CAD build for the part. Positions are in the model's coordinates, mm. Give positions to 0.01 mm unless a question says otherwise; leave off trailing zeros. Loops run counter-clockwise (first coordinate to the right, second up) from the corner with the lowest first, then second, coordinate; pieces in that order, holes last.
```python
from build123d import *

# Parameters (mm, degrees)
SKETCH_1_W             = 209.2
SKETCH_1_H             = 110
SM_BASE_FLANGE_1_DEPTH = 3.6
CUT_EXTRUDE_1_REACH    = 238.384
SKETCH_2_W             = 3.6
SKETCH_2_H             = 22
SKETCH_2_W_2           = 24
SKETCH_2_H_2           = 3.6
SKETCH_2_W_3           = 26
CUT_EXTRUDE_2_REACH    = 238.384
SKETCH_3_R             = 1.6


# Sheet-metal steps are written as plain solids
with BuildPart() as part:
    # Sketch 1 → Базовая кромка1 (new body)
    with BuildSketch(Plane.XY):
        with Locations((104.6, 55)):
            Rectangle(SKETCH_1_W, SKETCH_1_H)
    extrude(amount=-SM_BASE_FLANGE_1_DEPTH)

    # Sketch 2 → Вырез-Вытянуть1 (cut, up to next)
    with BuildSketch(Plane.XY, mode=Mode.PRIVATE) as cut_extrude_1_sk1:
        with Locations((1.8, 23)):
            Rectangle(SKETCH_2_W, SKETCH_2_H)
    cut_extrude_1_tool1 = extrude(cut_extrude_1_sk1.sketch, amount=-CUT_EXTRUDE_1_REACH, mode=Mode.PRIVATE) & part.part
    # Sketch 2 → Вырез-Вытянуть1 (cut, up to next)
    with BuildSketch(Plane.XY, mode=Mode.PRIVATE) as cut_extrude_1_sk2:
        with Locations((35.6, 1.8)):
            Rectangle(SKETCH_2_W_2, SKETCH_2_H_2)
    cut_extrude_1_tool2 = extrude(cut_extrude_1_sk2.sketch, amount=-CUT_EXTRUDE_1_REACH, mode=Mode.PRIVATE) & part.part
    # Sketch 2 → Вырез-Вытянуть1 (cut, up to next)
    with BuildSketch(Plane.XY, mode=Mode.PRIVATE) as cut_extrude_1_sk3:
        with Locations((207.4, 87)):
            Rectangle(SKETCH_2_W, SKETCH_2_H)
    cut_extrude_1_tool3 = extrude(cut_extrude_1_sk3.sketch, amount=-CUT_EXTRUDE_1_REACH, mode=Mode.PRIVATE) & part.part
    # Sketch 2 → Вырез-Вытянуть1 (cut, up to next)
    with BuildSketch(Plane.XY, mode=Mode.PRIVATE) as cut_extrude_1_sk4:
        with Locations((104.6, 1.8)):
            Rectangle(SKETCH_2_W_3, SKETCH_2_H_2)
    cut_extrude_1_tool4 = extrude(cut_extrude_1_sk4.sketch, amount=-CUT_EXTRUDE_1_REACH, mode=Mode.PRIVATE) & part.part
    # Sketch 2 → Вырез-Вытянуть1 (cut, up to next)
    with BuildSketch(Plane.XY, mode=Mode.PRIVATE) as cut_extrude_1_sk5:
        with Locations((173.6, 1.8)):
            Rectangle(SKETCH_2_W_2, SKETCH_2_H_2)
    cut_extrude_1_tool5 = extrude(cut_extrude_1_sk5.sketch, amount=-CUT_EXTRUDE_1_REACH, mode=Mode.PRIVATE) & part.part
    # Sketch 2 → Вырез-Вытянуть1 (cut, up to next)
    with BuildSketch(Plane.XY, mode=Mode.PRIVATE) as cut_extrude_1_sk6:
        with Locations((207.4, 23)):
            Rectangle(SKETCH_2_W, SKETCH_2_H)
    cut_extrude_1_tool6 = extrude(cut_extrude_1_sk6.sketch, amount=-CUT_EXTRUDE_1_REACH, mode=Mode.PRIVATE) & part.part
    # Sketch 2 → Вырез-Вытянуть1 (cut, up to next)
    with BuildSketch(Plane.XY, mode=Mode.PRIVATE) as cut_extrude_1_sk7:
        with Locations((173.6, 108.2)):
            Rectangle(SKETCH_2_W_2, SKETCH_2_H_2)
    cut_extrude_1_tool7 = extrude(cut_extrude_1_sk7.sketch, amount=-CUT_EXTRUDE_1_REACH, mode=Mode.PRIVATE) & part.part
    # Sketch 2 → Вырез-Вытянуть1 (cut, up to next)
    with BuildSketch(Plane.XY, mode=Mode.PRIVATE) as cut_extrude_1_sk8:
        with Locations((104.6, 108.2)):
            Rectangle(SKETCH_2_W_3, SKETCH_2_H_2)
    cut_extrude_1_tool8 = extrude(cut_extrude_1_sk8.sketch, amount=-CUT_EXTRUDE_1_REACH, mode=Mode.PRIVATE) & part.part
    # Sketch 2 → Вырез-Вытянуть1 (cut, up to next)
    with BuildSketch(Plane.XY, mode=Mode.PRIVATE) as cut_extrude_1_sk9:
        with Locations((35.6, 108.2)):
            Rectangle(SKETCH_2_W_2, SKETCH_2_H_2)
    cut_extrude_1_tool9 = extrude(cut_extrude_1_sk9.sketch, amount=-CUT_EXTRUDE_1_REACH, mode=Mode.PRIVATE) & part.part
    # Sketch 2 → Вырез-Вытянуть1 (cut, up to next)
    with BuildSketch(Plane.XY, mode=Mode.PRIVATE) as cut_extrude_1_sk10:
        with Locations((1.8, 87)):
            Rectangle(SKETCH_2_W, SKETCH_2_H)
    cut_extrude_1_tool10 = extrude(cut_extrude_1_sk10.sketch, amount=-CUT_EXTRUDE_1_REACH, mode=Mode.PRIVATE) & part.part
    add(cut_extrude_1_tool1.solids().sort_by_distance((1.8, 23, 0))[0], mode=Mode.SUBTRACT)
    add(cut_extrude_1_tool2.solids().sort_by_distance((35.6, 1.8, 0))[0], mode=Mode.SUBTRACT)
    add(cut_extrude_1_tool3.solids().sort_by_distance((207.4, 87, 0))[0], mode=Mode.SUBTRACT)
    add(cut_extrude_1_tool4.solids().sort_by_distance((104.6, 1.8, 0))[0], mode=Mode.SUBTRACT)
    add(cut_extrude_1_tool5.solids().sort_by_distance((173.6, 1.8, 0))[0], mode=Mode.SUBTRACT)
    add(cut_extrude_1_tool6.solids().sort_by_distance((207.4, 23, 0))[0], mode=Mode.SUBTRACT)
    add(cut_extrude_1_tool7.solids().sort_by_distance((173.6, 108.2, 0))[0], mode=Mode.SUBTRACT)
    add(cut_extrude_1_tool8.solids().sort_by_distance((104.6, 108.2, 0))[0], mode=Mode.SUBTRACT)
    add(cut_extrude_1_tool9.solids().sort_by_distance((35.6, 108.2, 0))[0], mode=Mode.SUBTRACT)
    add(cut_extrude_1_tool10.solids().sort_by_distance((1.8, 87, 0))[0], mode=Mode.SUBTRACT)

    # Эскиз3 → Вырез-Вытянуть2 (cut, up to next)
    with BuildSketch(Plane(origin=(0, 0, -3.6), x_dir=(-1, 0, 0), z_dir=(0, 0, -1)), mode=Mode.PRIVATE) as cut_extrude_2_sk1:
        with Locations((-9, 9)):
            Circle(SKETCH_3_R)
    cut_extrude_2_tool1 = extrude(cut_extrude_2_sk1.sketch, amount=-CUT_EXTRUDE_2_REACH, mode=Mode.PRIVATE) & part.part
    # Эскиз3 → Вырез-Вытянуть2 (cut, up to next)
    with BuildSketch(Plane(origin=(0, 0, -3.6), x_dir=(-1, 0, 0), z_dir=(0, 0, -1)), mode=Mode.PRIVATE) as cut_extrude_2_sk2:
        with Locations((-9, 101)):
            Circle(SKETCH_3_R)
    cut_extrude_2_tool2 = extrude(cut_extrude_2_sk2.sketch, amount=-CUT_EXTRUDE_2_REACH, mode=Mode.PRIVATE) & part.part
    # Эскиз3 → Вырез-Вытянуть2 (cut, up to next)
    with BuildSketch(Plane(origin=(0, 0, -3.6), x_dir=(-1, 0, 0), z_dir=(0, 0, -1)), mode=Mode.PRIVATE) as cut_extrude_2_sk3:
        with Locations((-200.2, 9)):
            Circle(SKETCH_3_R)
    cut_extrude_2_tool3 = extrude(cut_extrude_2_sk3.sketch, amount=-CUT_EXTRUDE_2_REACH, mode=Mode.PRIVATE) & part.part
    # Эскиз3 → Вырез-Вытянуть2 (cut, up to next)
    with BuildSketch(Plane(origin=(0, 0, -3.6), x_dir=(-1, 0, 0), z_dir=(0, 0, -1)), mode=Mode.PRIVATE) as cut_extrude_2_sk4:
        with Locations((-200.2, 101)):
            Circle(SKETCH_3_R)
    cut_extrude_2_tool4 = extrude(cut_extrude_2_sk4.sketch, amount=-CUT_EXTRUDE_2_REACH, mode=Mode.PRIVATE) & part.part
    add(cut_extrude_2_tool1.solids().sort_by_distance((9, 9, -3.6))[0], mode=Mode.SUBTRACT)
    add(cut_extrude_2_tool2.solids().sort_by_distance((9, 101, -3.6))[0], mode=Mode.SUBTRACT)
    add(cut_extrude_2_tool3.solids().sort_by_distance((200.2, 9, -3.6))[0], mode=Mode.SUBTRACT)
    add(cut_extrude_2_tool4.solids().sort_by_distance((200.2, 101, -3.6))[0], mode=Mode.SUBTRACT)


solid = part.part
```
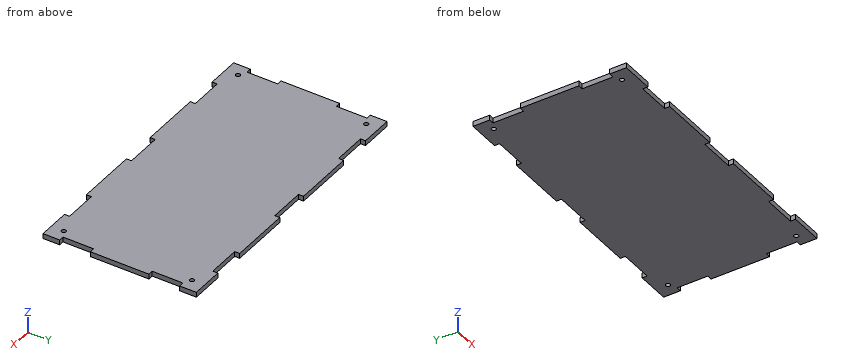
1. Saw through at C-C, the plane y = 20.5. List the corners of the cut face in (x, z), and give its area (3 significant figures).
Responses:
outline: (3.6, -3.6) - (205.6, -3.6) - (205.6, 0) - (3.6, 0) - close
area: 727 mm2
2. Saw through at B-B, the plane z = -0.75. Count the separate pieces of the cut face and the enclosed holes in it, and give its area (3 significant figures).
Responses:
separate pieces: 1
enclosed holes: 4
area: 22,100 mm2
3. Drop flat-ended pins along their axis: pin 1 (1 mm diameter, centred on y = 89, z = -2.5, fed in from +X); pin 2 (1.8 mm diameter, centred on y = 88.5, z = -1, fed in from -X). Give the stop position or say it passes through.
Responses:
pin 1: stops at x = 205.6
pin 2: stops at x = 3.6
4. Probe line 1 along Y through (x, z) = (9, -1.75); line 2 along X through (y, z) = (101, -1.4); line 3 along Y through (x, z) = (167, -2.65). List the from-to ranges inside material, lowest first.
Responses:
line 1: y = 0 to 7.4, 10.6 to 99.4, 102.6 to 110
line 2: x = 0 to 7.4, 10.6 to 198.6, 201.8 to 209.2
line 3: y = 3.6 to 106.4
5. Saw through at A-A, the plane x = 39. List the corners of the cut face in (y, z), and give its area (3 significant figures).
Responses:
outline: (3.6, -3.6) - (106.4, -3.6) - (106.4, 0) - (3.6, 0) - close
area: 370 mm2
